from build123d import *

# Parameters (mm, degrees)
SKETCH1_W           = 10.16
SKETCH1_H           = 10.16
BOSS_EXTRUDE1_DEPTH = 8.255
SKETCH2_W           = 3.556
SKETCH2_H           = 2.54
CUT_EXTRUDE3_DEPTH  = 10.16
CUT_EXTRUDE4_START  = -0.5715
SKETCH4_W           = 5.207
SKETCH4_H           = 5.461
CUT_EXTRUDE4_DEPTH  = 9.017
CUT_EXTRUDE5_START  = -0.5715
SKETCH5_W           = 5.334
SKETCH5_H           = 5.461
CUT_EXTRUDE5_DEPTH  = 9.017
SKETCH6_W           = 3.556
SKETCH6_H           = 2.54
CUT_EXTRUDE6_DEPTH  = 10.16
SKETCH7_W           = 5.207
SKETCH7_H           = 2.54
CUT_EXTRUDE7_DEPTH  = 10.16
SKETCH8_W           = 5.207
SKETCH8_H           = 2.54
CUT_EXTRUDE8_DEPTH  = 10.16


with BuildPart() as part:
    # Sketch1 → Boss-Extrude1 (new body)
    with BuildSketch(Plane(origin=(0, 0, 0), x_dir=(1, 0, 0), z_dir=(0, 1, 0))):
        with Locations((5.08, 5.08)):
            Rectangle(SKETCH1_W, SKETCH1_H)
    extrude(amount=BOSS_EXTRUDE1_DEPTH)

    # Sketch2 → Cut-Extrude3 (cut)
    with BuildSketch(Plane.XY):
        with Locations((5.08, 5.0165)):
            Rectangle(SKETCH2_W, SKETCH2_H)
    extrude(amount=-CUT_EXTRUDE3_DEPTH, mode=Mode.SUBTRACT)

    # Sketch4 → Cut-Extrude4 (cut)
    with BuildSketch(Plane.XY.offset(CUT_EXTRUDE4_START)):
        with Locations((5.08, 5.5245)):
            Rectangle(SKETCH4_W, SKETCH4_H)
    extrude(amount=-CUT_EXTRUDE4_DEPTH, mode=Mode.SUBTRACT)

    # Sketch5 → Cut-Extrude5 (cut)
    with BuildSketch(Plane(origin=(10.16, 0, 0), x_dir=(0, 0, -1), z_dir=(1, 0, 0)).offset(CUT_EXTRUDE5_START)):
        with Locations((5.0165, 5.5245)):
            Rectangle(SKETCH5_W, SKETCH5_H)
    extrude(amount=-CUT_EXTRUDE5_DEPTH, mode=Mode.SUBTRACT)

    # Sketch6 → Cut-Extrude6 (cut)
    with BuildSketch(Plane(origin=(10.16, 0, 0), x_dir=(0, 0, -1), z_dir=(1, 0, 0))):
        with Locations((5.08, 5.0165)):
            Rectangle(SKETCH6_W, SKETCH6_H)
    extrude(amount=-CUT_EXTRUDE6_DEPTH, mode=Mode.SUBTRACT)

    # Sketch7 → Cut-Extrude7 (cut)
    with BuildSketch(Plane.XY):
        with Locations((5.08, 5.0165)):
            Rectangle(SKETCH7_W, SKETCH7_H)
    extrude(amount=-CUT_EXTRUDE7_DEPTH, mode=Mode.SUBTRACT)

    # Sketch8 → Cut-Extrude8 (cut)
    with BuildSketch(Plane(origin=(10.16, 0, 0), x_dir=(0, 0, -1), z_dir=(1, 0, 0))):
        with Locations((5.08, 5.0165)):
            Rectangle(SKETCH8_W, SKETCH8_H)
    extrude(amount=-CUT_EXTRUDE8_DEPTH, mode=Mode.SUBTRACT)


solid = part.part
For this review, take the finished solid that the model builds, in its own axes (mm). A direction names the side the tool comes from. Give positions to 0.01 mm unless a question says otherwise; leave off trailing zeros. Loops run counter-clockwise (first coordinate to the right, second up) from the corner with the lowest first, then second, coordinate; pieces in that order, holes last.
Item 1: Take a section at B-B, the plane y = 3. State the section outline as (x, z) points, and give its area (3 significant figures).
Item 2: Take a section at A-A, the plane z = -5.25. State the section outline as (x, y) points (1 decimal).
Item 3: For line 1 along Z through (x, y) = (3.75, 7.75); line 2 along X through (y, z) = (7, -4); line 3 along Z through (x, y) = (9.25, 7), list the stretches that pass through material, from the lowest coordinate up.
Item 4: Take a section at C-C, the plane x = 7. State the section outline as (y, z) points (1 decimal).
Item 5: Insertion check: pin 1 (4.5 mm diameter, centred on x = 5, z = -6.5, fed in from +Y). The pin has a flat end and moves straight along its axis. Give the tip position at first contact, or say it passes through.
Item 6: Tool access review of faces 4 (the flat face through (10.16, 3, -5)), 5 (the flat face through (5, 3, -0.572)): name each direction out of +Z, -Z, +X, -X, +Y, -Y from which nothing blocks a thin tool from reaching the whole face with its end or side.
Item 7: Draft analysis for pull direction X (two halves, no side actions). For faces 1 (the flat face through (5, 3, 0)), 2 (the flat face through (0, 3, -5)), 3 (the flat face through (9.588, 7, -5)), state which applies: +X half, -X half, draft (parallel to the pull), parting line (faces both ways), or undercut.
Item 8: Take a section at D-D, the plane z = -8.25. State the section outline as (x, y) points (1 decimal), and give its area (3 significant figures).
Calculated:
1. outline: (0, -10.16) - (10.16, -10.16) - (10.16, 0) - (0, 0) - close; hole (0.57, -7.68) - (2.48, -7.68) - (2.48, -9.59) - (7.68, -9.59) - (7.68, -7.68) - (9.59, -7.68) - (9.59, -2.35) - (7.68, -2.35) - (7.68, -0.57) - (2.48, -0.57) - (2.48, -2.35) - (0.57, -2.35) - close
1. area: 36.0 mm2
2. outline: (0, 0) - (10.2, 0) - (10.2, 3.7) - (9.6, 3.7) - (9.6, 2.8) - (0.6, 2.8) - (0.6, 3.7) - (0, 3.7) - close; (0, 6.3) - (0.6, 6.3) - (0.6, 8.3) - (0, 8.3) - close; (9.6, 6.3) - (10.2, 6.3) - (10.2, 8.3) - (9.6, 8.3) - close
3. line 1: z = -10.16 to -9.59, -0.57 to 0
3. line 2: x = 0 to 0.57, 9.59 to 10.16
3. line 3: z = -10.16 to -7.68, -2.35 to 0
4. outline: (0, -10.2) - (3.7, -10.2) - (3.7, -9.6) - (2.8, -9.6) - (2.8, -0.6) - (3.7, -0.6) - (3.7, 0) - (0, 0) - close; (6.3, -10.2) - (8.3, -10.2) - (8.3, -9.6) - (6.3, -9.6) - close; (6.3, -0.6) - (8.3, -0.6) - (8.3, 0) - (6.3, 0) - close
5. pin 1: stops at y = 2.79
6. face 4: +Z, -Z, +X, +Y, -Y
6. face 5: +Y
7. face 1: draft
7. face 2: -X half
7. face 3: undercut
8. outline: (0, 0) - (10.2, 0) - (10.2, 8.3) - (7.7, 8.3) - (7.7, 2.8) - (2.5, 2.8) - (2.5, 8.3) - (0, 8.3) - close
8. area: 55.4 mm2
